For this review, take the finished solid that the model builds, in its own axes (mm). Face numbers are marked on the shaded views. A direction names the side the tool comes from. Coordinates: 2 decimals unless noted, no trailing zeros. Loops run counter-clockwise (first coordinate to the right, second up) from the corner with the lowest first, then second, coordinate; pieces in that order, holes last. Notation, with made-up numbers: M -31.5,70.25 L 26.5,70.25 A17 ccw 26.5,86.25 Z; hole C 17.25,71 d2. An arc over 180 degrees is marked long. Write each question's results on one line, items separated by ' | '. Start each with the question number.
```python
from build123d import *

# Parameters (mm, degrees)
SKETCH2_W           = 15.24
SKETCH2_H           = 15.24
BOSS_EXTRUDE1_DEPTH = 50.8
FILLET1_R           = 5.08
SKETCH4_W           = 40.555388052
SKETCH4_H           = 33.02
BOSS_EXTRUDE3_DEPTH = 25.4
SKETCH5_W           = 40.555388052
SKETCH5_H           = 21.336
CUT_EXTRUDE1_DEPTH  = 20.32
FILLET2_R           = 1.27
SKETCH3_R           = 11.43
BOSS_EXTRUDE2_DEPTH = 2.54


with BuildPart() as part:
    # Sketch1 → Revolve1 (revolve)
    with BuildSketch(Plane.XY):
        with BuildLine():
            Line((0, -15.875), (0, 15.875))
            ThreePointArc((0, 15.875), (15.875, 0), (0, -15.875))
        make_face()
    revolve(axis=Axis((0, -15.875, 0), (0, 1, 0)))

    # Sketch2 → Boss-Extrude1 (add)
    with BuildSketch(Plane(origin=(0, 0, 0), x_dir=(1, 0, 0), z_dir=(0, 1, 0))):
        Rectangle(SKETCH2_W, SKETCH2_H)
    extrude(amount=BOSS_EXTRUDE1_DEPTH)

    # Fillet1
    fillet1_edges = [part.edges().sort_by_distance(p)[0] for p in [
        (-7.62, 31.228525221, -7.62),
        (-7.62, 31.228525221, 7.62),
        (7.62, 31.228525221, 7.62),
        (7.62, 31.228525221, -7.62),
    ]]
    fillet(fillet1_edges, radius=FILLET1_R)

    # Sketch4 → Boss-Extrude3 (add)
    with BuildSketch(Plane(origin=(0, 50.8, 0), x_dir=(1, 0, 0), z_dir=(0, 1, 0))):
        Rectangle(SKETCH4_W, SKETCH4_H)
    extrude(amount=BOSS_EXTRUDE3_DEPTH)

    # Sketch5 → Cut-Extrude1 (cut)
    with BuildSketch(Plane(origin=(0, 76.2, 0), x_dir=(1, 0, 0), z_dir=(0, 1, 0))):
        Rectangle(SKETCH5_W, SKETCH5_H)
    extrude(amount=-CUT_EXTRUDE1_DEPTH, mode=Mode.SUBTRACT)

    # Fillet2
    fillet2_edges = [part.edges().sort_by_distance(p)[0] for p in [
        (-20.277694026, 50.8, 0),
        (-20.277694026, 63.5, -16.51),
        (0, 50.8, 16.51),
        (-20.277694026, 63.5, 16.51),
        (20.277694026, 50.8, 0),
        (20.277694026, 63.5, 16.51),
        (0, 50.8, -16.51),
        (20.277694026, 63.5, -16.51),
        (-20.277694026, 76.2, -13.589),
        (0, 76.2, 16.51),
        (0, 76.2, -16.51),
        (-20.277694026, 76.2, 13.589),
        (-20.277694026, 55.88, 0),
        (-20.277694026, 66.04, 10.668),
        (-20.277694026, 66.04, -10.668),
        (20.277694026, 55.88, 0),
        (20.277694026, 66.04, -10.668),
        (20.277694026, 66.04, 10.668),
    ]]
    fillet(fillet2_edges, radius=FILLET2_R)

    # Sketch3 → Boss-Extrude2 (add)
    with BuildSketch(Plane(origin=(0, 50.8, 0), x_dir=(1, 0, 0), z_dir=(0, 1, 0))):
        Circle(SKETCH3_R)
    extrude(amount=BOSS_EXTRUDE2_DEPTH)


solid = part.part
```
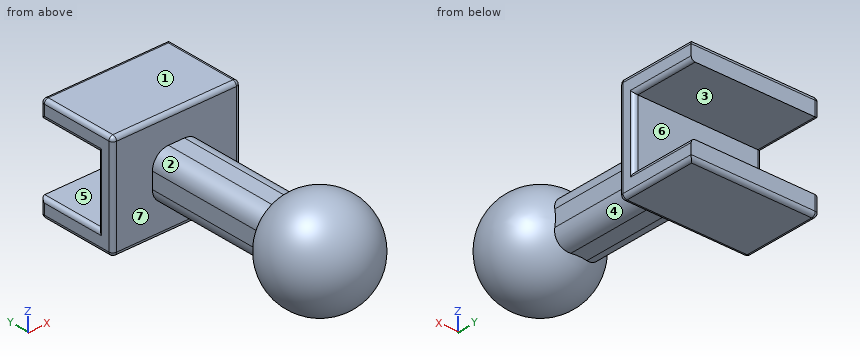
Q1. Take a section at B-B, the plane y = 67. Give the boundary of the cut face in (x, z).
Q2. The part is to be moulded in two halves that separate along Y. For the marked faces 5, 6 and 7, say which applies: pulls with the +Y half, pulls with the -Y half, needs draft (parallel to the pull), parting line crosses it, or undercut.
Q3. Take a section at D-D, the plane y = 16. Give the boundary of the cut face in (x, z).
Q4. Take a section at C-C, the plane x = -11. Give the boundary of the cut face in (y, z).
Q5. For the marked faces 1, 2, 3 and 4, list the 3-axis set-ups (+Z, -Z, +X, -X, +Y, -Y) from which the entire face can be reached by the end or side of a thin tool; tool diameter is ignored.
Q6. Insertion check: P1, Ø4, axis at y = 25, z = 0.5, coming from the +X side; P2, Ø10.5, axis at x = 1, z = -2.5, coming from the +Y side; P3, Ø1.5, axis at x = -8, y = 30, coming from the +Z side. Each pin has a flat end and moves straight along its axis. Give the tip position at first contact, or say it passes through.
Q7. To check wall thickness, follow line 1 along Z through (x, y) = (-11, 56); line 2 along X through (y, z) = (34.5, 2); line 3 along Y through (x, z) = (-11, -2). State the ranges of each line that lie inside material, in increasing order.
Q8. Take a section at A-A, the plane z = 9.5. Give the boundary of the cut face in (x, y).
Results:
1) outline: M -20.28,-15.24 A1.27 ccw -19.01,-16.51 L 19.01,-16.51 A1.27 ccw 20.28,-15.24 L 20.28,-11.94 A1.27 ccw 19.01,-10.67 L -19.01,-10.67 A1.27 ccw -20.28,-11.94 Z; M -20.28,11.94 A1.27 ccw -19.01,10.67 L 19.01,10.67 A1.27 ccw 20.28,11.94 L 20.28,15.24 A1.27 ccw 19.01,16.51 L -19.01,16.51 A1.27 ccw -20.28,15.24 Z
2) face 5: needs draft | face 6: pulls with the +Y half | face 7: undercut
3) outline: M -7.62,-2.54 A5.08 ccw -2.54,-7.62 L 2.54,-7.62 A5.08 ccw 7.62,-2.54 L 7.62,2.54 A5.08 ccw 2.54,7.62 L -2.54,7.62 A5.08 ccw -7.62,2.54 Z
4) outline: C 0,0 d22.89; M 50.8,-15.24 A1.27 ccw 52.07,-16.51 L 74.93,-16.51 A1.27 ccw 76.2,-15.24 L 76.2,-10.67 L 55.88,-10.67 L 55.88,10.67 L 76.2,10.67 L 76.2,15.24 A1.27 ccw 74.93,16.51 L 52.07,16.51 A1.27 ccw 50.8,15.24 Z
5) face 1: +Z, +X, -X, +Y, -Y | face 2: +Z, -X | face 3: +X, -X, +Y | face 4: -Z, +X
6) P1: x = 7.62 | P2: y = 55.88 | P3: z = 4.44
7) line 1: -16.51 to -10.67, 10.67 to 16.51 | line 2: -7.62 to 7.62 | line 3: -11.27 to 11.27, 50.8 to 55.88
8) outline: M -20.28,52.07 A1.27 ccw -19.01,50.8 L 19.01,50.8 A1.27 ccw 20.28,52.07 L 20.28,54.61 A1.27 ccw 19.01,55.88 L -19.01,55.88 A1.27 ccw -20.28,54.61 Z; C 0,0 d25.44
